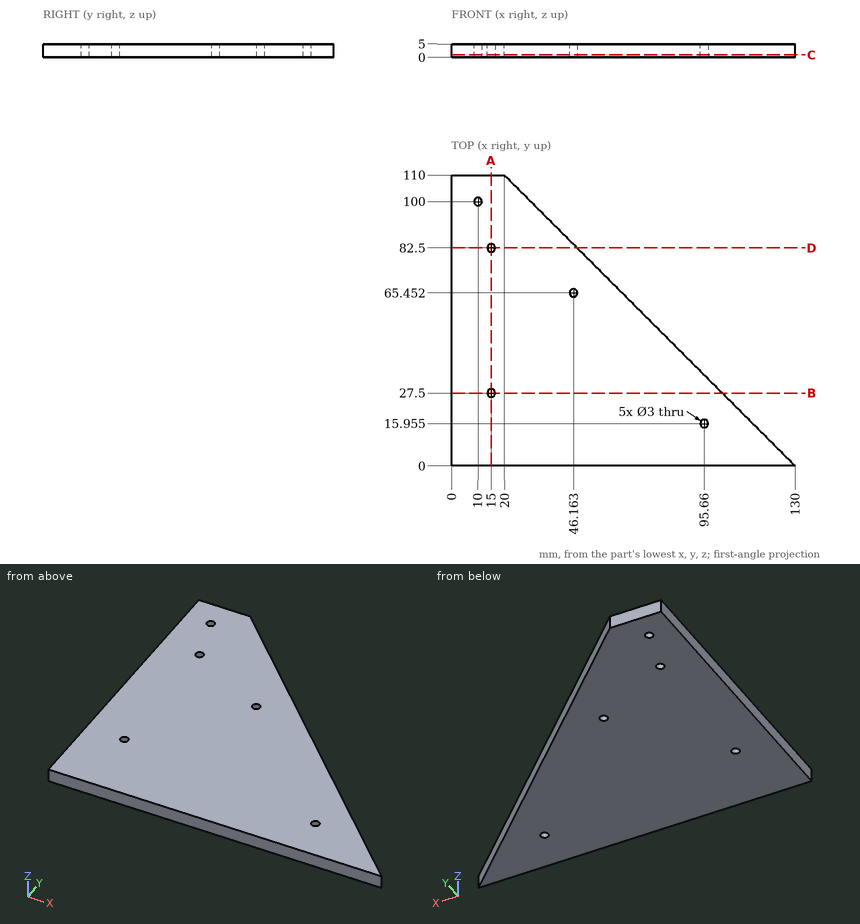
Geometry: see drawing. Coordinates: mm, zero at the bounding-box minimum. Coordinates: 2 decimals unless noted, no trailing zeros. Order: outer loops, then holes, each group sorted by start corner. A loop starts at its lowest first (then second) coordinate and runs counter-clockwise, first axis right, second up. Notation, with made-up numbers: (0, -34.5) - (55, -34.5) arc R13 ccw to (55, -30.5) - close; hole circle Ø4 at (70, 82.5). An arc over 180 degrees is marked (long way). Write each question's results on one line, items separated by ' | '.
1) Section B-B, the plane y = 27.5. Return loops of the section in (x, z).
Results list:
outline: (0, 0) - (13.5, 0) - (13.5, 5) - (0, 5) - close; (16.5, 0) - (102.5, 0) - (102.5, 5) - (16.5, 5) - close
2) Section A-A, the plane x = 15. Return loops of the section in (y, z), plus the area to 3 significant figures.
Results list:
outline: (0, 0) - (26, 0) - (26, 5) - (0, 5) - close; (29, 0) - (81, 0) - (81, 5) - (29, 5) - close; (84, 0) - (110, 0) - (110, 5) - (84, 5) - close | area: 520 mm^2
3) Line query: line 1 (Y direction, x = 15, z = 3); line 2 (Y direction, x = 14, z = 1.15); line 3 (Y direction, x = 10, z = 1.35). Output: solid intervals per line, ascending. Write a range as from..to.
Results list:
line 1: 0..26, 29..81, 84..110 | line 2: 0..26.38, 28.62..81.38, 83.62..110 | line 3: 0..98.5, 101.5..110
4) Section C-C, the plane z = 0.85. Return loops of the section in (x, y) (1 decimal).
Results list:
outline: (0, 0) - (130, 0) - (20, 110) - (0, 110) - close; hole circle Ø3 at (10, 100); hole circle Ø3 at (15, 27.5); hole circle Ø3 at (15, 82.5); hole circle Ø3 at (46.2, 65.5); hole circle Ø3 at (95.7, 16)
5) Section D-D, the plane y = 82.5. Return loops of the section in (x, z).
Results list:
outline: (0, 0) - (13.5, 0) - (13.5, 5) - (0, 5) - close; (16.5, 0) - (47.5, 0) - (47.5, 5) - (16.5, 5) - close
